Verification items for the finished model (mm, model axes). Give positions to 0.01 mm unless a question says otherwise; leave off trailing zeros. Order: outer loops, then holes, each group sorted by start corner. A loop starts at its lowest first (then second) coordinate and runs counter-clockwise, first axis right, second up.
from build123d import *

# Parameters (mm, degrees)
BOSS_EXTRUDE1_DEPTH      = 3
CUT_EXTRUDE2_DEPTH       = 295.638673234
CUT_EXTRUDE2_DEPTH_BACK  = 3
CUT_EXTRUDE6_DEPTH       = 295.638673234
CUT_EXTRUDE6_DEPTH_BACK  = 3
CUT_EXTRUDE11_DEPTH      = 295.638673234
CUT_EXTRUDE11_DEPTH_BACK = 3
CUT_EXTRUDE12_DEPTH      = 295.638673234
CUT_EXTRUDE12_DEPTH_BACK = 3
SKETCH9_W                = 3
SKETCH9_H                = 30
CUT_EXTRUDE13_DEPTH      = 3
SKETCH10_W               = 2.5
SKETCH10_H               = 42
CUT_EXTRUDE14_DEPTH      = 10
SKETCH11_R               = 1.5
CUT_EXTRUDE15_DEPTH      = 10


with BuildPart() as part:
    # Sketch1 → Boss-Extrude1 (new body)
    with BuildSketch(Plane(origin=(0, 0, 0), x_dir=(0, 0, -1), z_dir=(1, 0, 0))):
        Polygon((286.144320394, 0.17389594), (286.144320394, 70.17389594), (-16.855679606, 70.17389594), (-116.855679606, 40.17389594), (-119.855679606, 40.17389594), (-119.855679606, 0.17389594), align=None)
    extrude(amount=BOSS_EXTRUDE1_DEPTH)

    # Sketch5 → Cut-Extrude2 (cut, two sides: drawn at the far end of the back side and taken through both)
    with BuildSketch(Plane(origin=(3, 0, 0), x_dir=(0, 0, -1), z_dir=(1, 0, 0)).offset(-CUT_EXTRUDE2_DEPTH_BACK)):
        Polygon((1115.56118622, 55.17389594), (286.144320394, 55.17389594), (283.144320394, 55.17389594), (283.144320394, 15.17389594), (286.144320394, 15.17389594), (1115.56118622, 15.17389594), (2774.394917872, 15.17389594), (2774.394917872, 55.17389594), align=None)
    extrude(amount=CUT_EXTRUDE2_DEPTH + CUT_EXTRUDE2_DEPTH_BACK, mode=Mode.SUBTRACT)

    # Sketch6 → Cut-Extrude6 (cut, two sides: drawn at the far end of the back side and taken through both)
    with BuildSketch(Plane(origin=(3, 0, 0), x_dir=(0, 0, -1), z_dir=(1, 0, 0)).offset(-CUT_EXTRUDE6_DEPTH_BACK)):
        Polygon((253.144320394, 839.196952243), (253.144320394, 70.17389594), (253.144320394, 67.17389594), (13.144320394, 67.17389594), (13.144320394, 70.17389594), (13.144320394, 839.196952243), (13.144320394, 2377.24306485), (253.144320394, 2377.24306485), align=None)
    extrude(amount=CUT_EXTRUDE6_DEPTH + CUT_EXTRUDE6_DEPTH_BACK, mode=Mode.SUBTRACT)

    # Sketch7 → Cut-Extrude11 (cut, two sides: drawn at the far end of the back side and taken through both)
    with BuildSketch(Plane(origin=(3, 0, 0), x_dir=(0, 0, -1), z_dir=(1, 0, 0)).offset(-CUT_EXTRUDE11_DEPTH_BACK)):
        Polygon((-264.146282978, 799.817128167), (-42.908554564, 62.358033452), (-42.046510907, 59.484554597), (-89.937825168, 45.117160318), (-90.799868825, 47.990639174), (-312.037597239, 785.449733889), (-754.513054068, 2260.367923318), (-706.621739807, 2274.735317597), align=None)
    extrude(amount=CUT_EXTRUDE11_DEPTH + CUT_EXTRUDE11_DEPTH_BACK, mode=Mode.SUBTRACT)

    # Sketch8 → Cut-Extrude12 (cut, two sides: drawn at the far end of the back side and taken through both)
    with BuildSketch(Plane(origin=(3, 0, 0), x_dir=(0, 0, -1), z_dir=(1, 0, 0)).offset(-CUT_EXTRUDE12_DEPTH_BACK)):
        Polygon((-950.674782697, 30.17389594), (-119.855679606, 30.17389594), (-116.855679606, 30.17389594), (-116.855679606, 10.17389594), (-119.855679606, 10.17389594), (-950.674782697, 10.17389594), (-2612.31298888, 10.17389594), (-2612.31298888, 30.17389594), align=None)
    extrude(amount=CUT_EXTRUDE12_DEPTH + CUT_EXTRUDE12_DEPTH_BACK, mode=Mode.SUBTRACT)

    # Sketch9 → Cut-Extrude13 (cut)
    with BuildSketch(Plane(origin=(3, 0, 0), x_dir=(0, 0, -1), z_dir=(1, 0, 0))):
        with Locations((-15.355679606, 35.17389594)):
            Rectangle(SKETCH9_W, SKETCH9_H)
    extrude(amount=-CUT_EXTRUDE13_DEPTH, mode=Mode.SUBTRACT)

    # Sketch10 → Cut-Extrude14 (cut)
    with BuildSketch(Plane(origin=(3, 0, 0), x_dir=(0, 0, -1), z_dir=(1, 0, 0))):
        with Locations((19.894320394, 36.17389594)):
            Rectangle(SKETCH10_W, SKETCH10_H)
    extrude(amount=-CUT_EXTRUDE14_DEPTH, mode=Mode.SUBTRACT)

    # Sketch11 → Cut-Extrude15 (cut)
    with BuildSketch(Plane(origin=(3, 0, 0), x_dir=(0, 0, -1), z_dir=(1, 0, 0))):
        with Locations((236.144320394, 3.17389594)):
            Circle(SKETCH11_R)
        with Locations((86.144320394, 3.17389594)):
            Circle(SKETCH11_R)
        with Locations((-63.855679606, 3.17389594)):
            Circle(SKETCH11_R)
    extrude(amount=-CUT_EXTRUDE15_DEPTH, mode=Mode.SUBTRACT)


solid = part.part
(1) Go/stop test with flat-tipped pins: pin 1 (1.5 mm diameter, centred on x = 2.5, z = -179, fed in from +Y); pin 2 (1 mm diameter, centred on x = 2.5, y = 38.5, fed in from -Z); pin 3 (1.8 mm diameter, centred on y = 3.17, z = -236.14, fed in from -X). Record where each tip stops, or that it passes through.
Solved:
pin 1: stops at y = 67.17
pin 2: stops at z = -283.14
pin 3: passes through
(2) Section check A-A, the plane y = 35. Enter the section's corners in (x, z), then the cut area to 3 significant figures.
Solved:
outline: (0, -283.14) - (3, -283.14) - (3, -21.14) - (0, -21.14) - close; (0, -18.64) - (3, -18.64) - (3, 13.86) - (0, 13.86) - close; (0, 16.86) - (3, 16.86) - (3, 119.86) - (0, 119.86) - close
area: 1,190 mm2
(3) Section check D-D, the plane z = 75.5. Enter the section's corners in (x, y), then the cut area to 3 significant figures.
Solved:
outline: (0, 0.17) - (3, 0.17) - (3, 49.45) - (0, 49.45) - close
area: 148 mm2
(4) Section check B-B, the plane x = 1.1. Give the number of separate pieces and of enclosed holes in the cut face, then the cut area to 3 significant figures.
Solved:
separate pieces: 1
enclosed holes: 5
area: 25,600 mm2
(5) Scan lines: line 1 (Z direction, x = 0.85, y = 33); line 2 (Z direction, x = 2.4, y = 27); line 3 (Z direction, x = 1.05, y = 19). Record each from-to range of solid material in increasing order.
Solved:
line 1: z = -283.14 to -21.14, -18.64 to 13.86, 16.86 to 119.86
line 2: z = -283.14 to -21.14, -18.64 to 13.86, 16.86 to 116.86
line 3: z = -283.14 to -21.14, -18.64 to 116.86
(6) Section check C-C, the plane z = -72. Enter the section's corners in (x, y), then the cut area to 3 significant figures.
Solved:
outline: (0, 0.17) - (3, 0.17) - (3, 67.17) - (0, 67.17) - close
area: 201 mm2
